The listing builds one solid part. Answer for the finished solid, in the listing's coordinates (mm). Face numbers are marked on the shaded views. A direction names the side the tool comes from. Give positions to 0.01 mm unless a question says otherwise; leave off trailing zeros. Order: outer loops, then holes, each group sorted by start corner. A loop starts at its lowest first (then second) coordinate and runs counter-clockwise, first axis right, second up. Notation, with made-up numbers: (75.25, 10.5) - (126.25, 10.5) arc R6 ccw to (126.25, 18.5) - close; hole circle Ø8 at (79.25, 56.25). An arc over 180 degrees is marked (long way). Answer as CSV lines item,"result". Start each with the question number.
1. Section C-C on x = 322.5 is taken. Give the vertices of the cut face in (y, z).
2. Section A-A on x = 204.5 is taken. Give the vertices of the cut face in (y, z).
3. Determine the mould class of the marked faces 3, 4 and 5 for opening direction Z: +Z half, -Z half, draft (parallel to the pull), parting line (faces both ways), or undercut.
4. Consider line 1 along Z through (x, y) = (296.5, -32.5); line 2 along X through (y, z) = (-18, -74); line 3 along Y through (x, z) = (272, -171). Determine where each line is inside the solid, lowest interval first. Write a range as [from, to].
5. Section B-B on z = -264 is taken. Give the vertices of the cut face in (x, y).
6. Flat-ended cylindrical pins translate along their axes: pin 1 (1.2 mm diameter, centred on x = 343.5, y = 3.5, fed in from +Z); pin 2 (1.5 mm diameter, centred on y = -32.5, z = -43, fed in from +X); pin 3 (2 mm diameter, centred on x = 324.5, z = -57, fed in from +Y). Find the tip coordinate at first contact, or state that the pin passes through.
7. Which of the six approach directions +Z, -Z, +X, -X, +Y, -Y give full straight-line access (tool end or side, diameter ignored) to the marked faces 1 and 2?
from build123d import *

# Parameters (mm, degrees)
BOSS_EXTRUDE4_DEPTH  = 1.5
SKETCH5_W            = 155
SKETCH5_H            = 54
BOSS_EXTRUDE5_DEPTH  = 1.5
SKETCH8_W            = 1.5
SKETCH8_H            = 330
BOSS_EXTRUDE14_DEPTH = 4
SKETCH7_W            = 155
SKETCH7_H            = 54
BOSS_EXTRUDE18_DEPTH = 1.5
SKETCH9_W            = 333
SKETCH9_H            = 54
BOSS_EXTRUDE19_DEPTH = 1.5


with BuildPart() as part:
    # Sketch4 → Boss-Extrude4 (new body)
    with BuildSketch(Plane(origin=(0, 0, 0), x_dir=(1, 0, 0), z_dir=(0, 1, 0))):
        Polygon((189.373653762, 330), (344.373653762, 330), (344.373653762, 0), (189.373653762, 0), (189.373653762, 65), (231.373653762, 65), (231.373653762, 130), (189.373653762, 130), align=None)
    extrude(amount=BOSS_EXTRUDE4_DEPTH)

    # Sketch5 → Boss-Extrude5 (add)
    with BuildSketch(Plane.XY):
        with Locations((266.873653762, -25.5)):
            Rectangle(SKETCH5_W, SKETCH5_H)
    extrude(amount=BOSS_EXTRUDE5_DEPTH)

    # Sketch8 → Boss-Extrude14 (add)
    with BuildSketch(Plane(origin=(0, 1.5, 0), x_dir=(1, 0, 0), z_dir=(0, 1, 0))):
        with Locations((343.623653762, 165)):
            Rectangle(SKETCH8_W, SKETCH8_H)
    extrude(amount=BOSS_EXTRUDE14_DEPTH)

    # Sketch7 → Boss-Extrude18 (add)
    with BuildSketch(Plane(origin=(0, 0, -330), x_dir=(-1, 0, 0), z_dir=(0, 0, -1))):
        with Locations((-266.873653762, -25.5)):
            Rectangle(SKETCH7_W, SKETCH7_H)
    extrude(amount=BOSS_EXTRUDE18_DEPTH)

    # Sketch9 → Boss-Extrude19 (add)
    with BuildSketch(Plane.ZY.offset(-189.373653762)):
        with Locations((-165, -25.5)):
            Rectangle(SKETCH9_W, SKETCH9_H)
    extrude(amount=BOSS_EXTRUDE19_DEPTH)


solid = part.part
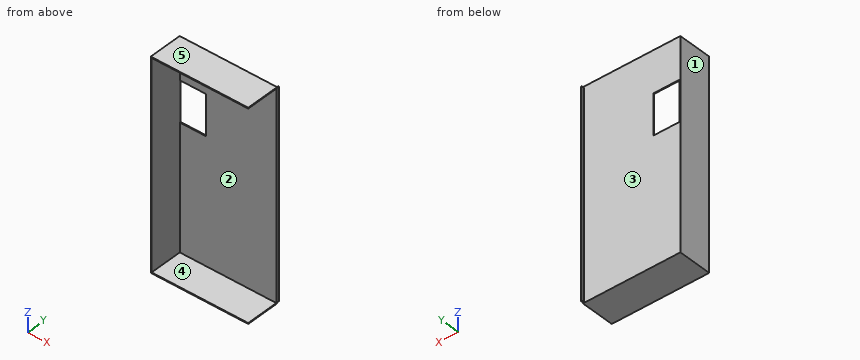
Checks:
1,outline,"(-52.5, -331.5) - (1.5, -331.5) - (1.5, 1.5) - (-52.5, 1.5) - (-52.5, 0) - (0, 0) - (0, -330) - (-52.5, -330) - close"
2,outline,"(-52.5, -331.5) - (1.5, -331.5) - (1.5, -130) - (0, -130) - (0, -330) - (-52.5, -330) - close; (-52.5, 0) - (0, 0) - (0, -65) - (1.5, -65) - (1.5, 1.5) - (-52.5, 1.5) - close"
3,face 3,"draft"
3,face 4,"undercut"
3,face 5,"+Z half"
4,line 1,"z = [-331.5, -330], [0, 1.5]"
4,line 2,"x = [187.87, 189.37]"
4,line 3,"y = [0, 1.5]"
5,outline,"(187.87, -52.5) - (189.37, -52.5) - (189.37, 0) - (344.37, 0) - (344.37, 5.5) - (342.87, 5.5) - (342.87, 1.5) - (187.87, 1.5) - close"
6,pin 1,"stops at z = 0"
6,pin 2,"stops at x = 189.37"
6,pin 3,"stops at y = 1.5"
7,face 1,"+Z, -Z, -X, +Y, -Y"
7,face 2,"+X, -Y"
